from build123d import *

# Parameters (mm, degrees)
SKETCH1_W           = 38.1
SKETCH1_H           = 50.8
BOSS_EXTRUDE1_DEPTH = 3.175
SKETCH2_W           = 3.048
SKETCH2_H           = 50.8
BOSS_EXTRUDE2_DEPTH = 19.05
SKETCH3_R           = 1.75
CUT_EXTRUDE1_DEPTH  = 38.026544532
SKETCH4_R           = 1.75
CUT_EXTRUDE2_DEPTH  = 42.305517564


with BuildPart() as part:
    # Sketch1 → Boss-Extrude1 (new body)
    with BuildSketch(Plane(origin=(0, 0, 0), x_dir=(1, 0, 0), z_dir=(0, 1, 0))):
        Rectangle(SKETCH1_W, SKETCH1_H)
    extrude(amount=BOSS_EXTRUDE1_DEPTH)

    # Sketch2 → Boss-Extrude2 (add)
    with BuildSketch(Plane(origin=(0, 3.175, 0), x_dir=(1, 0, 0), z_dir=(0, 1, 0))):
        with Locations((-3.2385, 0)):
            Rectangle(SKETCH2_W, SKETCH2_H)
        with Locations((3.1115, 0)):
            Rectangle(SKETCH2_W, SKETCH2_H)
    extrude(amount=BOSS_EXTRUDE2_DEPTH)

    # Sketch3 → Cut-Extrude1 (cut, through all)
    with BuildSketch(Plane(origin=(0, 3.175, 0), x_dir=(1, 0, 0), z_dir=(0, 1, 0))):
        with Locations(Location((-12.7, 19.05, 0), (0, 0, 270))):
            Circle(SKETCH3_R)
        with Locations(Location((-12.7, -19.05, 0), (0, 0, 270))):
            Circle(SKETCH3_R)
        with Locations(Location((12.7, -19.05, 0), (0, 0, 270))):
            Circle(SKETCH3_R)
        with Locations(Location((12.7, 19.05, 0), (0, 0, 270))):
            Circle(SKETCH3_R)
    extrude(amount=-CUT_EXTRUDE1_DEPTH, mode=Mode.SUBTRACT)

    # Sketch4 → Cut-Extrude2 (cut, through all)
    with BuildSketch(Plane.ZY.offset(4.7625)):
        with Locations((-16.51, 13.612832847)):
            Circle(SKETCH4_R)
        with Locations((16.51, 13.612832847)):
            Circle(SKETCH4_R)
    extrude(amount=-CUT_EXTRUDE2_DEPTH, mode=Mode.SUBTRACT)


solid = part.part
Could you check a few things on this model? Use its own coordinates, in mm. A direction names the side the tool comes from. Give positions to 0.01 mm unless a question says otherwise; leave off trailing zeros. Order: outer loops, then holes, each group sorted by start corner. A loop starts at its lowest first (then second) coordinate and runs counter-clockwise, first axis right, second up. Notation, with made-up numbers: (-39.75, 6.5) - (-14.75, 6.5) arc R22 ccw to (-14.75, 35.5) - close; hole circle Ø4 at (47, 57.25). An arc over 180 degrees is marked (long way). Return JSON: item names as keys, results as strings. Group by question number.
Q1. Suppose I cut it at B-B, the plane z = 19.05. State how many separate pieces and enclosed holes the cut face has, and give its area (3 significant figures).
Q2. Thinking about a two-plate mould opening in Z: for faces 6 (the face through (19.05, 2, 0)), 7 (the face through (-11.224, 1.61, -18.109)), 8 (the face through (-3, 8, -25.4)), which applies, pulls with the +Z half, pulls with the -Z half, needs draft (parallel to the pull), parting line crosses it, or undercut?
Q3. Which directions (+Z, -Z, +X, -X, +Y, -Y) give clear straight access to the entire face, cutting with the end or side of a thin tool? Please do faces 1 (the face through (13.226, 1.61, -17.381)), 2 (the face through (-3.26, 12.55, 15.12)), 3 (the face through (-1.715, 13, 0)), 4 (the face through (-12, 3.175, 0)), 5 (the face through (12, 3.175, 0)).
Q4. Suppose I cut it at C-C, the plane x = -12.7. Please give me the cut outline in (y, z) (3 decimals).
Q5. Will these pins go through, and if not, where does the flat tip stop? pin 1 Ø2 at (y, z) = (18.5, -9) entering from -X; pin 2 Ø4.5 at (x, z) = (-11.5, -1.5) entering from +Y (3 decimals); pin 3 Ø12 at (y, z) = (7, -3.5) entering from +X; pin 4 Ø4.5 at (y, z) = (13.61, 16.51) entering from +X.
Q6. Please list where these lines run through material, in increasing order: line 1 along X through (y, z) = (1.05, 19.05); line 2 along X through (y, z) = (14.5, 20); line 3 along Y through (x, z) = (2.9, -16.51) (3 decimals). Write a range as [from, to].
Q7. Suppose I cut it at A-A, the plane y = 9.25. Please give me the cut outline in (x, z), and give its area (3 significant figures).
Resolved:
{
 "1": {"separate pieces": "3", "enclosed holes": "0", "area": "215 mm2"},
 "2": {"face 6": "needs draft", "face 7": "undercut", "face 8": "pulls with the -Z half"},
 "3": {"face 1": "+Y, -Y", "face 2": "+X, -X", "face 3": "+Z, -Z, +Y", "face 4": "+Z, -Z, -X, +Y", "face 5": "+Z, -Z, +X, +Y"},
 "4": {"outline": "(0, -25.4) - (3.175, -25.4) - (3.175, -20.8) - (0, -20.8) - close; (0, -17.3) - (3.175, -17.3) - (3.175, 17.3) - (0, 17.3) - close; (0, 20.8) - (3.175, 20.8) - (3.175, 25.4) - (0, 25.4) - close"},
 "5": {"pin 1": "stops at x = -4.76", "pin 2": "stops at y = 3.175", "pin 3": "stops at x = 19.05", "pin 4": "stops at x = 4.64"},
 "6": {"line 1": "x = [-19.05, -14.45], [-10.95, 10.95], [14.45, 19.05]", "line 2": "x = [-4.76, -1.71], [1.59, 4.64]", "line 3": "y = [0, 11.863], [15.363, 22.225]"},
 "7": {"outline": "(-4.76, -25.4) - (-1.71, -25.4) - (-1.71, 25.4) - (-4.76, 25.4) - close; (1.59, -25.4) - (4.64, -25.4) - (4.64, 25.4) - (1.59, 25.4) - close", "area": "310 mm2"}
}
